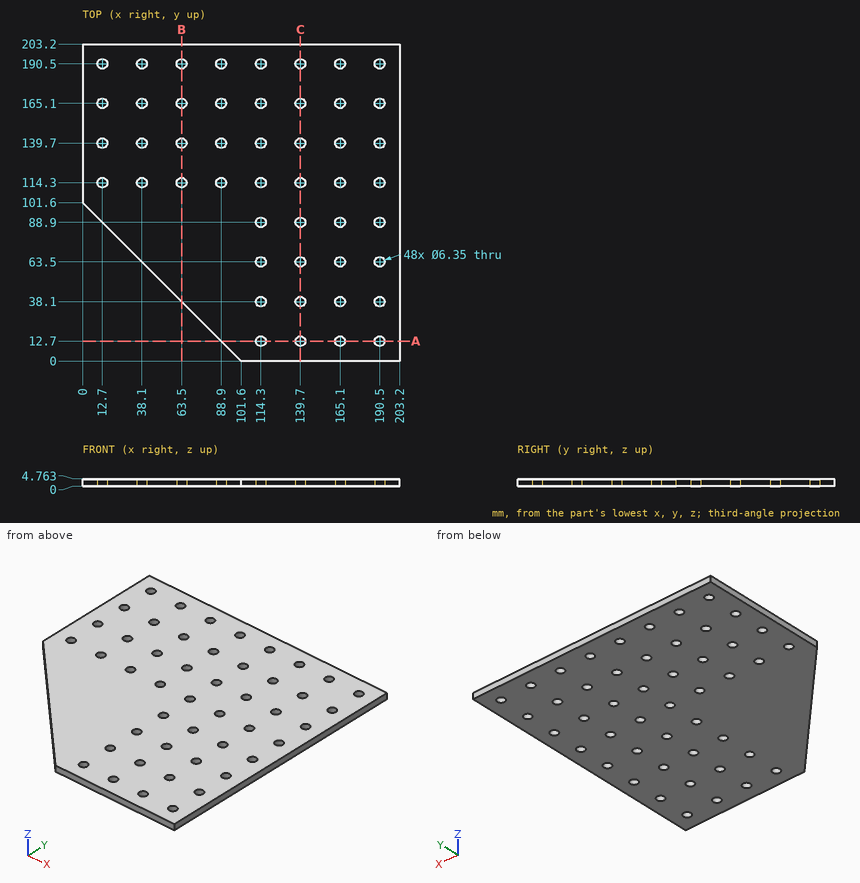
Check sheet for the drawn part. Datum: minimum x, y, z corner. Units: mm. Round coordinates to 2 decimals unless told otherwise and drop trailing zeros. Write each loop counter-clockwise with the first axis right and the second up, starting at its lowest first coordinate (ties: lowest second). Pieces come first, ordered by that corner, then holes. Notation, with made-up numbers: (39, 54.5) -> (53, 54.5) arc R34 ccw to (53, 90.5) -> close; hole circle Ø2 at (79, -16.75). An arc over 180 degrees is marked (long way). Put each result on its own line as item: value.
(1) Material ranges on line 1 (X direction, y = 15.5, z = 1.85) (1 decimal); line 2 (X direction, y = 88.9, z = 1.65) (1 decimal); line 3 (Y direction, x = 39.5, z = 0.95), recorded low to high.
Values found:
line 1: x = 86.1 to 112.8, 115.8 to 138.2, 141.2 to 163.6, 166.6 to 189, 192 to 203.2
line 2: x = 12.7 to 111.1, 117.5 to 136.5, 142.9 to 161.9, 168.3 to 187.3, 193.7 to 203.2
line 3: y = 62.1 to 111.45, 117.15 to 136.85, 142.55 to 162.25, 167.95 to 187.65, 193.35 to 203.2
(2) Sectioned sample at A-A (y = 12.7). Enter the section's corners in (x, z) (1 decimal).
Values found:
outline: (88.9, 0) -> (111.1, 0) -> (111.1, 4.8) -> (88.9, 4.8) -> close; (117.5, 0) -> (136.5, 0) -> (136.5, 4.8) -> (117.5, 4.8) -> close; (142.9, 0) -> (161.9, 0) -> (161.9, 4.8) -> (142.9, 4.8) -> close; (168.3, 0) -> (187.3, 0) -> (187.3, 4.8) -> (168.3, 4.8) -> close; (193.7, 0) -> (203.2, 0) -> (203.2, 4.8) -> (193.7, 4.8) -> close
(3) Go/stop test with flat-tipped pins: pin 1 Ø10 at (x, y) = (190.5, 38.1) entering from -Z; pin 2 Ø5.5 at (x, y) = (114.3, 190.5) entering from -Z. Record where each tip stops, or that it passes through.
Values found:
pin 1: stops at z = 0
pin 2: passes through
(4) Sectioned sample at B-B (x = 63.5). Enter the section's corners in (y, z) (1 decimal).
Values found:
outline: (38.1, 0) -> (111.1, 0) -> (111.1, 4.8) -> (38.1, 4.8) -> close; (117.5, 0) -> (136.5, 0) -> (136.5, 4.8) -> (117.5, 4.8) -> close; (142.9, 0) -> (161.9, 0) -> (161.9, 4.8) -> (142.9, 4.8) -> close; (168.3, 0) -> (187.3, 0) -> (187.3, 4.8) -> (168.3, 4.8) -> close; (193.7, 0) -> (203.2, 0) -> (203.2, 4.8) -> (193.7, 4.8) -> close
(5) Sectioned sample at C-C (x = 139.7). Count the separate pieces of the cut face and the enclosed holes in it.
Values found:
separate pieces: 9
enclosed holes: 0
